from build123d import *

# Parameters (mm, degrees)
SKETCH1_R           = 11.5
SKETCH1_R_2         = 10
BOSS_EXTRUDE1_DEPTH = 10
SKETCH2_R           = 11.5
SKETCH2_R_2         = 10
SKETCH2_R_3         = 5.558376586
BOSS_EXTRUDE3_DEPTH = 2
SKETCH2_3_R         = 5.558376586
SKETCH2_3_R_2       = 4.575743436
BOSS_EXTRUDE4_DEPTH = 10
SKETCH3_R           = 5.558376586
BOSS_EXTRUDE5_DEPTH = 2
CUT_EXTRUDE1_DEPTH  = 8


with BuildPart() as part:
    # Sketch1 → Boss-Extrude1 (new body)
    with BuildSketch(Plane(origin=(0, 0, 0), x_dir=(1, 0, 0), z_dir=(0, 1, 0))):
        Circle(SKETCH1_R)
        Circle(SKETCH1_R_2, mode=Mode.SUBTRACT)
    extrude(amount=BOSS_EXTRUDE1_DEPTH)

    # Sketch2 → Boss-Extrude3 (add)
    with BuildSketch(Plane.XZ):
        Circle(SKETCH2_R)
        Circle(SKETCH2_R_2, mode=Mode.SUBTRACT)
        Circle(SKETCH2_R_2)
        Circle(SKETCH2_R_3, mode=Mode.SUBTRACT)
    extrude(amount=BOSS_EXTRUDE3_DEPTH)

    # Sketch2_3 → Boss-Extrude4 (add)
    with BuildSketch(Plane.XZ):
        Circle(SKETCH2_3_R)
        Circle(SKETCH2_3_R_2, mode=Mode.SUBTRACT)
    extrude(amount=BOSS_EXTRUDE4_DEPTH)

    # Sketch3 → Boss-Extrude5 (add)
    with BuildSketch(Plane.XZ.offset(10)):
        Circle(SKETCH3_R)
    extrude(amount=BOSS_EXTRUDE5_DEPTH)

    # Sketch4 → Cut-Extrude1 (cut)
    with BuildSketch(Plane(origin=(0, 10, 0), x_dir=(1, 0, 0), z_dir=(0, 1, 0))):
        with BuildLine():
            Line((-5.820799865, -9.918078893), (-5.0615651, -8.624416429))
            ThreePointArc((-5.0615651, -8.624416429), (-0.071235745, -9.99974627), (4.93818117, -8.695652174))
            Line((4.93818117, -8.695652174), (5.678908346, -10))
            ThreePointArc((5.678908346, -10), (-0.081921107, -11.499708211), (-5.820799865, -9.918078893))
        make_face()
        with BuildLine():
            Line((-5.678908346, 10), (-4.93818117, 8.695652174))
            ThreePointArc((-4.93818117, 8.695652174), (-8.624416429, 5.0615651), (-9.99974627, 0.071235745))
            Line((-9.99974627, 0.071235745), (-11.499708211, 0.081921107))
            ThreePointArc((-11.499708211, 0.081921107), (-9.918078893, 5.820799865), (-5.678908346, 10))
        make_face()
        with BuildLine():
            Line((11.499708211, -0.081921107), (9.99974627, -0.071235745))
            ThreePointArc((9.99974627, -0.071235745), (8.695652174, 4.93818117), (5.0615651, 8.624416429))
            Line((5.0615651, 8.624416429), (5.820799865, 9.918078893))
            ThreePointArc((5.820799865, 9.918078893), (10, 5.678908346), (11.499708211, -0.081921107))
        make_face()
    extrude(amount=-CUT_EXTRUDE1_DEPTH, mode=Mode.SUBTRACT)


solid = part.part
The model under review builds one solid part; all positions refer to its coordinate system, in mm. A direction names the side the tool comes from. Coordinates: 2 decimals unless noted, no trailing zeros. Write each loop counter-clockwise with the first axis right and the second up, starting at its lowest first coordinate (ties: lowest second). Pieces come first, ordered by that corner, then holes. Notation, with made-up numbers: (-0.5, -11.75) - (16.5, -11.75) arc R18 cw to (16.5, 4.25) - close; hole circle Ø10 at (-18.5, -36.75). An arc over 180 degrees is marked (long way). Answer as a JSON object with one key per item and string values. Group by question number.
1. Mouldability with a two-part tool opening along X and no side actions: class faces 5 (the face through (0, -10, 0)), 6 (the face through (-5.314, 6.056, -9.357)), 7 (the face through (-5.553, -6.93, 0.244)) as pulls with the +X half, pulls with the -X half, needs draft (parallel to the pull), parting line crosses it, or undercut.
2. Add section B-B (x = 0). Give the boundary of the cut face in (y, z), plus the area to 3 significant figures.
3. Add section D-D (y = -2.5). Give the boundary of the cut face in (x, z).
4. Add section A-A (y = 8.25). Give the boundary of the cut face in (x, z), plus the area to 3 significant figures.
5. Clearance check with flat-ended pins moving along their axes: pin 1 Ø2.5 at (x, z) = (-2, 10.5) entering from +Y; pin 2 Ø6 at (x, z) = (-4, -2.5) entering from +Y; pin 3 Ø4 at (x, y) = (-8, 0) entering from +Z; pin 4 Ø4 at (x, y) = (-9, -9.5) entering from +Z. State where each tip first meets the part, or that it passes through.
6. Machinability: for faces 1 (the face through (5.303, 6.056, 9.339)), 2 (the face through (4.3, 0, -2.1)), 3 (the face through (5, -2, 3)), 4 (the face through (5.436, 6.056, -9.262)), which of the approach directions +Z, -Z, +X, -X, +Y, -Y give a long, thin tool a straight path to every point of the face, cutting with its end or side? Answer none if there is none.
7. Add section C-C (z = -6.5). Give the boundary of the cut face in (x, y), plus the area to 3 significant figures.
8. To check wall thickness, follow probe 1 along Z at (x, y) = (0, -4); probe 2 along Y at (x, z) = (-1.75, 4); probe 3 along Y at (x, z) = (3.75, 6.25). State the ranges of each line that lie inside material, in increasing order.
Findings:
{
 "1": {"face 5": "undercut", "face 6": "pulls with the -X half", "face 7": "parting line crosses it"},
 "2": {"outline": "(-12, -5.56) - (-2, -5.56) - (-2, -11.5) - (10, -11.5) - (10, -10) - (0, -10) - (0, -4.58) - (-10, -4.58) - (-10, 4.58) - (0, 4.58) - (0, 10) - (2, 10) - (2, 11.5) - (-2, 11.5) - (-2, 5.56) - (-12, 5.56) - close", "area": "83.7 mm²"},
 "3": {"outline": "circle Ø11.12 at (0, 0); hole circle Ø9.15 at (0, 0)"},
 "4": {"outline": "(-11.5, -0.08) - (-10, -0.07) arc R10 cw to (-5.06, 8.62) - (-5.82, 9.92) arc R11.5 ccw to start; (-5.68, -10) arc R11.5 ccw to (5.82, -9.92) - (5.06, -8.62) arc R10 cw to (-4.94, -8.7) - close; (4.94, 8.7) arc R10 cw to (10, 0.07) - (11.5, 0.08) arc R11.5 ccw to (5.68, 10) - close", "area": "50.7 mm²"},
 "5": {"pin 1": "y = 2", "pin 2": "y = 0", "pin 3": "z = 9.81", "pin 4": "through"},
 "6": {"face 1": "+Z, +Y", "face 2": "+Y", "face 3": "-Y", "face 4": "+X, +Y"},
 "7": {"outline": "(-9.49, -2) - (9.49, -2) - (9.49, 2) - (7.6, 2) - (7.6, 0) - (-7.6, 0) - (-7.6, 2) - (-9.49, 2) - close", "area": "45.5 mm²"},
 "8": {"probe 1": "-5.56 to -4.58, 4.58 to 5.56", "probe 2": "-12 to -10", "probe 3": "-2 to 0"}
}
